The model under review builds one solid part; all positions refer to its coordinate system, in mm. Round coordinates to 2 decimals unless told otherwise and drop trailing zeros. Order: outer loops, then holes, each group sorted by start corner. A loop starts at its lowest first (then second) coordinate and runs counter-clockwise, first axis right, second up. Notation, with made-up numbers: M 31.5,7 L 41.5,7 A12 cw 41.5,11 Z; hole C 21.25,3 d10. An arc over 180 degrees is marked long. Answer as a JSON object with one key per item and string values. Group by question number.
1) Consider section A-A, the plane z = 0. Write out the cut boundary in (x, y), then the cut area to 3 significant figures.
2) Consider section B-B, the plane y = 12.5. Write out the cut boundary in (x, z).
3) Consider section D-D, the plane y = 22. Write out the cut boundary in (x, z), then the cut area to 3 significant figures.
4) Insertion check: pin 1 Ø2.5 at (y, z) = (12.5, 0) entering from +X. The pin has a flat end and moves straight along its axis. Give the tip position at first contact, or say it passes through.
5) The part is to be moulded in two halves that separate along Z. For faces 1 (the cylindrical face through (8, 11, 0)), 2 (the flat face through (-13, 12, -2)), 3 (the cylindrical face through (12.14, 12.32, 7.1)), say which applies: +Z half, -Z half, draft (parallel to the pull), parting line (faces both ways), or undercut.
6) To check wall thickness, follow line 1 (Y direction, x = -10, z = 0); line 2 (Z direction, x = 6.5, y = 12.5); line 3 (X direction, y = 10, z = 0). State the ranges of each line that lie inside material, in increasing order.
7) Consider section C-C, the plane x = 0. Write out the cut boundary in (y, z).
```python
from build123d import *

# Parameters (mm, degrees)
SKETCH1_R           = 4
BOSS_EXTRUDE1_DEPTH = 25
SKETCH2_R           = 1.5
CUT_EXTRUDE1_DEPTH  = 46


with BuildPart() as part:
    # Sketch1 → Boss-Extrude1 (new body)
    with BuildSketch(Plane(origin=(0, 0, 0), x_dir=(1, 0, 0), z_dir=(0, 1, 0))):
        with BuildLine():
            Line((10, -8), (-10, -8))
            ThreePointArc((-10, -8), (-12.121320344, -7.121320344), (-13, -5))
            Line((-13, -5), (-13, 5))
            ThreePointArc((-13, 5), (-12.121320344, 7.121320344), (-10, 8))
            Line((-10, 8), (10, 8))
            ThreePointArc((10, 8), (12.121320344, 7.121320344), (13, 5))
            Line((13, 5), (13, -5))
            ThreePointArc((13, -5), (12.121320344, -7.121320344), (10, -8))
        make_face()
        with Locations(Location((0, 0, 0), (0, 0, 270))):
            Circle(SKETCH1_R, mode=Mode.SUBTRACT)
    extrude(amount=BOSS_EXTRUDE1_DEPTH)

    # Sketch2 → Cut-Extrude1 (cut)
    with BuildSketch(Plane(origin=(13, 0, 0), x_dir=(0, 0, -1), z_dir=(1, 0, 0))):
        with Locations((0, 12.5)):
            Circle(SKETCH2_R)
    extrude(amount=-CUT_EXTRUDE1_DEPTH, mode=Mode.SUBTRACT)


solid = part.part
```
Results list:
{
 "1": {"outline": "M -13,0 L -4,0 L -4,11 L -13,11 Z; M -13,14 L -4,14 L -4,25 L -13,25 Z; M 4,0 L 13,0 L 13,11 L 4,11 Z; M 4,14 L 13,14 L 13,25 L 4,25 Z", "area": "396 mm^2"},
 "2": {"outline": "M -13,-5 A3 ccw -10,-8 L 10,-8 A3 ccw 13,-5 L 13,-1.5 L 3.71,-1.5 A4 cw -3.71,-1.5 L -13,-1.5 Z; M -13,1.5 L -3.71,1.5 A4 cw 3.71,1.5 L 13,1.5 L 13,5 A3 ccw 10,8 L -10,8 A3 ccw -13,5 Z"},
 "3": {"outline": "M -13,-5 A3 ccw -10,-8 L 10,-8 A3 ccw 13,-5 L 13,5 A3 ccw 10,8 L -10,8 A3 ccw -13,5 Z; hole C 0,0 d8", "area": "358 mm^2"},
 "4": {"pin 1": "through"},
 "5": {"face 1": "undercut", "face 2": "draft", "face 3": "+Z half"},
 "6": {"line 1": "0 to 11, 14 to 25", "line 2": "-8 to -1.5, 1.5 to 8", "line 3": "-13 to -4, 4 to 13"},
 "7": {"outline": "M 0,-8 L 25,-8 L 25,-4 L 0,-4 Z; M 0,4 L 25,4 L 25,8 L 0,8 Z"}
}
